Work out the finished part from the listing and answer in its coordinate system (mm). Face numbers are marked on the shaded views. A direction names the side the tool comes from. Coordinates: 2 decimals unless noted, no trailing zeros. Write each loop counter-clockwise with the first axis right and the second up, starting at its lowest first coordinate (ties: lowest second). Pieces come first, ordered by that corner, then holes. Notation, with made-up numbers: (76, 39) - (86, 39) arc R7 ccw to (86, 45) - close; hole circle Ø10 at (61.5, -17). An arc over 180 degrees is marked (long way). Use a Markdown table: item, result. Add a question column.
(1) The part is cut by section B-B, the plane y = -27. Give the vertices of the cut face in (x, z), then the cut area to 3 significant figures.
(2) The part is cut by section D-D, the plane y = 1.5. Give the vertices of the cut face in (x, z), then the cut area to 3 significant figures.
(3) The part is cut by section A-A, the plane z = 7. Give the vertices of the cut face in (x, y), then the cut area to 3 significant figures.
(4) For a pull along Y with two mould halves and no side action, classify the marked faces 1, 2, 3 and 4 as released by +Y, released by -Y, zero draft, split by the parting line, or undercut.
(5) Find the intervals of material crossed by line 1 (Y direction, x = -48, z = 2); line 2 (X direction, y = 28.5, z = 1.25); line 3 (Y direction, x = 46, z = 3), in increasing order. Write a range as from..to.
(6) Given pin 1 Ø17.5 at (x, y) = (-36, -11.5) entering from +Z; pin 2 Ø1.5 at (y, z) = (-9.5, 11.5) entering from +X, each flat-ended and moving along its own axis, determine where each tip first touches the part or whether it passes through.
(7) The part is cut by section C-C, the plane x = -51.5. Give the vertices of the cut face in (y, z).
(8) A tool of negligible diameter and unlimited length cuts with its end or side. For the marked faces 5, 6 and 7, from which of +Z, -Z, +X, -X, +Y, -Y can it reach the whole face along a straight path? Write none if from no direction.
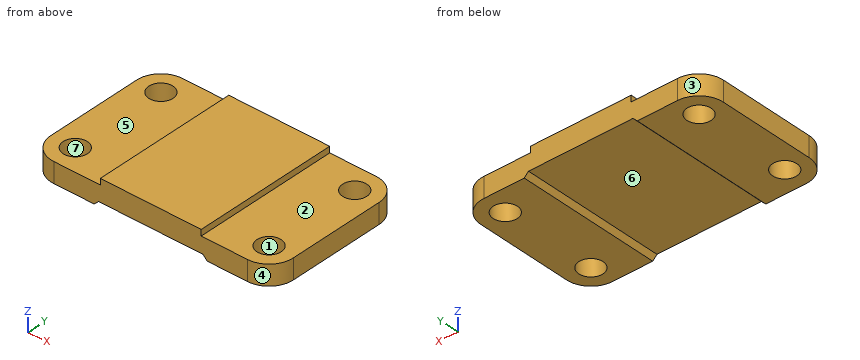
from build123d import *

# Parameters (mm, degrees)
BOSS_EXTRUDE1_DEPTH = 10
SKETCH2_R           = 6
CUT_EXTRUDE1_DEPTH  = 71.682388188
CUT_EXTRUDE2_DEPTH  = 95.254973344
SKETCH4_W           = 50
SKETCH4_H           = 72
BOSS_EXTRUDE2_DEPTH = 3


with BuildPart() as part:
    # Sketch1 → Boss-Extrude1 (new body)
    with BuildSketch(Plane.XY):
        with BuildLine():
            Line((-48, 36), (48, 36))
            ThreePointArc((48, 36), (56.485281374, 32.485281374), (60, 24))
            Line((60, 24), (60, -24))
            ThreePointArc((60, -24), (56.485281374, -32.485281374), (48, -36))
            Line((48, -36), (-48, -36))
            ThreePointArc((-48, -36), (-56.485281374, -32.485281374), (-60, -24))
            Line((-60, -24), (-60, 24))
            ThreePointArc((-60, 24), (-56.485281374, 32.485281374), (-48, 36))
        make_face()
    extrude(amount=BOSS_EXTRUDE1_DEPTH)

    # Sketch2 → Cut-Extrude1 (cut, through all)
    with BuildSketch(Plane.XY.offset(10)):
        with Locations((-48, 24)):
            Circle(SKETCH2_R)
        with Locations((-48, -24)):
            Circle(SKETCH2_R)
        with Locations(Location((48, -24, 0), (0, 0, 180))):
            Circle(SKETCH2_R)
        with Locations(Location((48, 24, 0), (0, 0, 180))):
            Circle(SKETCH2_R)
    extrude(amount=-CUT_EXTRUDE1_DEPTH, mode=Mode.SUBTRACT)

    # Sketch3 → Cut-Extrude2 (cut, through all)
    with BuildSketch(Plane.XZ.offset(36)):
        Polygon((-28, 0), (28, 0), (25.878679656, 2.121320344), (-25.878679656, 2.121320344), align=None)
    extrude(amount=-CUT_EXTRUDE2_DEPTH, mode=Mode.SUBTRACT)

    # Sketch4 → Boss-Extrude2 (add)
    with BuildSketch(Plane.XY.offset(10)):
        Rectangle(SKETCH4_W, SKETCH4_H)
    extrude(amount=BOSS_EXTRUDE2_DEPTH)


solid = part.part
Model answer:
| question | item | result |
|---|---|---|
| 1 | outline | (-59.62, 0) - (-53.2, 0) - (-53.2, 10) - (-59.62, 10) - close; (-42.8, 0) - (-28, 0) - (-25.88, 2.12) - (25.88, 2.12) - (28, 0) - (42.8, 0) - (42.8, 10) - (25, 10) - (25, 13) - (-25, 13) - (-25, 10) - (-42.8, 10) - close; (53.2, 0) - (59.62, 0) - (59.62, 10) - (53.2, 10) - close |
| 1 | area | 1,020 mm^2 |
| 2 | outline | (-60, 0) - (-28, 0) - (-25.88, 2.12) - (25.88, 2.12) - (28, 0) - (60, 0) - (60, 10) - (25, 10) - (25, 13) - (-25, 13) - (-25, 10) - (-60, 10) - close |
| 2 | area | 1,240 mm^2 |
| 3 | outline | (-60, -24) arc R12 ccw to (-48, -36) - (48, -36) arc R12 ccw to (60, -24) - (60, 24) arc R12 ccw to (48, 36) - (-48, 36) arc R12 ccw to (-60, 24) - close; hole circle Ø12 at (-48, -24); hole circle Ø12 at (-48, 24); hole circle Ø12 at (48, -24); hole circle Ø12 at (48, 24) |
| 3 | area | 8,060 mm^2 |
| 4 | face 1 | undercut |
| 4 | face 2 | zero draft |
| 4 | face 3 | released by +Y |
| 4 | face 4 | released by -Y |
| 5 | line 1 | -36..-30, -18..18, 30..36 |
| 5 | line 2 | -59.12..-51.97, -44.03..-26.75, 26.75..44.03, 51.97..59.12 |
| 5 | line 3 | -36..-29.66, -18.34..18.34, 29.66..36 |
| 6 | pin 1 | z = 10 |
| 6 | pin 2 | x = 25 |
| 7 | outline | (-35.48, 0) - (-28.87, 0) - (-28.87, 10) - (-35.48, 10) - close; (-19.13, 0) - (19.13, 0) - (19.13, 10) - (-19.13, 10) - close; (28.87, 0) - (35.48, 0) - (35.48, 10) - (28.87, 10) - close |
| 8 | face 5 | +Z, -X, +Y, -Y |
| 8 | face 6 | -Z, +Y, -Y |
| 8 | face 7 | +Z, -Z |
